Here's how the part is built. I have some questions about the finished solid (model axes, mm). Round coordinates to 2 decimals unless told otherwise and drop trailing zeros. Write each loop counter-clockwise with the first axis right and the second up, starting at its lowest first coordinate (ties: lowest second). Pieces come first, ordered by that corner, then holes. Notation, with made-up numbers: (35.5, 27.25) -> (69.5, 27.25) arc R19 cw to (69.5, 57.25) -> close; hole circle Ø7 at (-10, -3). An arc over 180 degrees is marked (long way). Answer as CSV lines item,"result".
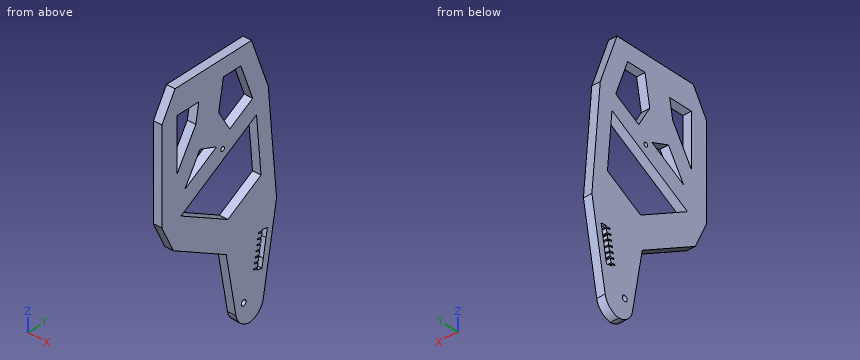
```python
from build123d import *

# Parameters (mm, degrees)
ESQUISSE1_W                             = 300
ESQUISSE1_H                             = 150
BOSS_EXTRU_1_DEPTH                      = 5
ESQUISSE2_OUTSIDE_W                     = 369.112
ESQUISSE2_OUTSIDE_H                     = 219.112
ENL_V_MAT_EXTRU_1_DEPTH                 = 5
ENL_V_MAT_EXTRU_2_DEPTH                 = 336.559234711
ENL_V_MAT_EXTRU_2_DEPTH_BACK            = 336.559234711
ENL_V_MAT_EXTRU_4_DEPTH                 = 336.559234711
ENL_V_MAT_EXTRU_4_DEPTH_BACK            = 336.559234711
ESQUISSE5_R                             = 3.2
EMPREINTE1_START                        = -213.565883238
EMPREINTE1_OUTLINE_W                    = 10
EMPREINTE1_OUTLINE_H                    = 6
EMPREINTE1_DEPTH                        = 20
D_PLACER_START                          = -213.815883238
D_PLACER_LA_FACE1_OUTLINE_W             = 10
D_PLACER_LA_FACE1_OUTLINE_H             = 6.5
D_PLACER_LA_FACE1_DEPTH                 = 20.5
D_PLACER_LA_FACE2_BY                    = 10
D_PLACER_LA_FACE3_BY                    = 10
ENL_V_MAT_EXTRU_5_DEPTH                 = 336.559234711
R_P_TITION_LIN_AIRE1_COUNT              = 7
R_P_TITION_LIN_AIRE1_PITCH              = 6
CONG_1_R                                = 20
PER_AGE_POUR_CROUS_AUTO_BLOQUANTS_300_D = 4.7625


# Read off the part's stored shape, not the designer's step: Empreinte1, Déplacer la face1
with BuildPart() as part:
    # Esquisse1 → Boss.-Extru.1 (new, symmetric)
    with BuildSketch(Plane(origin=(0, 0, 0), x_dir=(0, 0, -1), z_dir=(1, 0, 0))):
        with Locations((150, 75)):
            Rectangle(ESQUISSE1_W, ESQUISSE1_H)
    extrude(amount=BOSS_EXTRU_1_DEPTH, both=True)

    # Esquisse2 outside → Enlèv. mat.-Extru.1 (cut, symmetric)
    with BuildSketch(Plane(origin=(0, 0, 0), x_dir=(0, 0, -1), z_dir=(1, 0, 0))):
        with Locations((150, 75)):
            Rectangle(ESQUISSE2_OUTSIDE_W, ESQUISSE2_OUTSIDE_H)
        Polygon((0, 117.225703003), (60, 139.063917059), (185, 150), (300, 129.722397219), (300, 99.722397219), (211.741963761, 84.160124165), (171.741963761, 14.878091862), (139.835792798, 0), (29.835792798, 0), (0, 17.225703003), align=None, mode=Mode.SUBTRACT)
    extrude(amount=ENL_V_MAT_EXTRU_1_DEPTH, both=True, mode=Mode.SUBTRACT)

    # Esquisse3 → Enlèv. mat.-Extru.2 (cut, two sides: drawn at the far end of the back side and taken through both)
    with BuildSketch(Plane(origin=(5, 0, 0), x_dir=(0, 0, -1), z_dir=(1, 0, 0)).offset(-ENL_V_MAT_EXTRU_2_DEPTH_BACK)):
        Polygon((20, 103.221552239), (20, 80.493304508), (55, 74.321860183), (80, 88.755616913), (62.679491924, 118.755616913), align=None)
        Polygon((90, 71.435108837), (113.922571241, 30), (81.508057782, 49.831775443), align=None)
        Polygon((82.886751346, 123.755616913), (139.903333355, 25), (175.32640016, 86.354551467), (150.32640016, 129.655821657), align=None)
        Polygon((91.944969354, 20), (30, 20), (30, 48.267236345), (52.117107943, 44.367393479), align=None)
    extrude(amount=ENL_V_MAT_EXTRU_2_DEPTH + ENL_V_MAT_EXTRU_2_DEPTH_BACK, mode=Mode.SUBTRACT)

    # Esquisse5 → Enlèv. mat.-Extru.4 (cut, two sides: drawn at the far end of the back side and taken through both)
    with BuildSketch(Plane.ZY.offset(5).offset(-ENL_V_MAT_EXTRU_4_DEPTH_BACK)):
        with Locations((-275, 107.010571736)):
            Circle(ESQUISSE5_R)
    extrude(amount=ENL_V_MAT_EXTRU_4_DEPTH + ENL_V_MAT_EXTRU_4_DEPTH_BACK, mode=Mode.SUBTRACT)

    # Empreinte1 outline → Empreinte1 (cut)
    with BuildSketch(Plane(origin=(0, 0, 0), x_dir=(1, 0, 0), z_dir=(0, 0.173648177666931, 0.984807753012208)).offset(EMPREINTE1_START)):
        with Locations((0, 169.157749671)):
            Rectangle(EMPREINTE1_OUTLINE_W, EMPREINTE1_OUTLINE_H)
    extrude(amount=EMPREINTE1_DEPTH, mode=Mode.SUBTRACT)

    # Déplacer la face1 outline → Déplacer la face1 (cut)
    with BuildSketch(Plane(origin=(0, 0, 0), x_dir=(1, 0, 0), z_dir=(0, 0.173648177666931, 0.984807753012208)).offset(D_PLACER_START)):
        with Locations((0, 169.157749671)):
            Rectangle(D_PLACER_LA_FACE1_OUTLINE_W, D_PLACER_LA_FACE1_OUTLINE_H)
    extrude(amount=D_PLACER_LA_FACE1_DEPTH, mode=Mode.SUBTRACT)

    # Déplacer la face2: a face moved inward by 10.0
    extrude(part.faces().sort_by_distance((0, 133.01891252, -219.752915562))[0], amount=D_PLACER_LA_FACE2_BY, dir=(0, 0.173648178, 0.984807753), mode=Mode.SUBTRACT)

    # Déplacer la face3: a face moved inward by 10.0
    extrude(part.faces().sort_by_distance((0, 129.459124878, -239.941474499))[0], amount=D_PLACER_LA_FACE3_BY, dir=(0, -0.173648178, -0.984807753), mode=Mode.SUBTRACT)

    # Esquisse6 → Enlèv. mat.-Extru.5 (cut, through all)
    with BuildSketch(Plane(origin=(5, 0, 0), x_dir=(0, 0, -1), z_dir=(1, 0, 0))):
        Polygon((210.817693083, 131.294296833), (209.949452195, 126.370258067), (211.328183049, 126.127150619), (212.196423938, 131.051189384), align=None)
    enl_v_mat_extru_5 = extrude(amount=-ENL_V_MAT_EXTRU_5_DEPTH, mode=Mode.SUBTRACT)

    # Répétition linéaire1: Enlèv. mat.-Extru.5 ×7
    with Locations(*[Vector(0, -0.17364817766693066, -0.9848077530122081) * (i * R_P_TITION_LIN_AIRE1_PITCH) for i in range(1, R_P_TITION_LIN_AIRE1_COUNT)]):
        add(enl_v_mat_extru_5, mode=Mode.SUBTRACT)

    # Congé1
    # the kernel refuses this fillet: 20 mm, written as the material it takes off along each edge
    with BuildSketch(Plane(origin=(-46.954981559, 129.722397219, -300), x_dir=(0, 0.17364817766693125, 0.9848077530122079), z_dir=(1, 0, 0))) as cong_1_piece_1:
        with BuildLine():
            CenterArc((CONG_1_R * 0.839099631177, CONG_1_R), CONG_1_R, 190, 80)
            Line((-CONG_1_R * 0.145708121835, CONG_1_R * 0.826351822333), (0, 0))
            Line((0, 0), (CONG_1_R * 0.839099631177, 0))
        make_face()
    extrude(amount=93.909963118, mode=Mode.SUBTRACT)
    with BuildSketch(Plane(origin=(-46.954981559, 99.722397219, -300), x_dir=(0, -0.17364817766692434, 0.984807753012209), z_dir=(1, 0, 0))) as cong_1_piece_2:
        with BuildLine():
            CenterArc((CONG_1_R * 0.839099631177, -CONG_1_R), CONG_1_R, 90, 80)
            Line((-CONG_1_R * 0.145708121835, -CONG_1_R * 0.826351822333), (0, 0))
            Line((0, 0), (CONG_1_R * 0.839099631177, 0))
        make_face()
    extrude(amount=93.909963118, mode=Mode.SUBTRACT)

    # Perçage pour écrous auto-bloquants 300® #6 (SP)1 (through all)
    with Locations(Plane(origin=(5, 0, 0), x_dir=(0, 0, -1), z_dir=(1, 0, 0))):
        with Locations((96.461753504, 79.36920384)):
            Hole(PER_AGE_POUR_CROUS_AUTO_BLOQUANTS_300_D / 2)


solid = part.part
```
1. For pin 1 Ø1 at (x, z) = (2, -70.5) entering from -Y; pin 2 Ø5 at (x, z) = (1, -75.5) entering from +Y; pin 3 Ø1 at (x, z) = (-3.5, -136) entering from +Y, each with a flat end and sliding along its axis, tell me the tip position at first contact or that it passes through.
Numbers:
pin 1,"stops at y = 0"
pin 2,"stops at y = 140.64"
pin 3,"stops at y = 145.76"
2. Suppose I cut it at C-C on y = 38. Please give me the cut outline in (x, z), and give its area (3 significant figures).
Numbers:
outline,"(-5, -185.09) -> (5, -185.09) -> (5, -147.41) -> (-5, -147.41) -> close; (-5, -132.4) -> (5, -132.4) -> (5, -109.3) -> (-5, -109.3) -> close; (-5, -100.85) -> (5, -100.85) -> (5, -62.52) -> (-5, -62.52) -> close; (-5, -30) -> (5, -30) -> (5, 0) -> (-5, 0) -> close"
area,"1,290 mm^2"
3. Suppose I cut it at A-A on z = -275. Please give me the cut outline in (x, y).
Numbers:
outline,"(-5, 95.31) -> (5, 95.31) -> (5, 103.81) -> (-5, 103.81) -> close; (-5, 110.21) -> (5, 110.21) -> (5, 134.13) -> (-5, 134.13) -> close"
4. If I drill on line 1 (Z direction, x = -2, y = 53); line 2 (Z direction, x = -0.25, y = 98.5); line 3 (Y direction, x = 3, z = -231.5), over which ranges is the centre line in solid material (lowest first)?
Numbers:
line 1,"z = -193.75 to -156.07, -123.74 to -100.64, -82.75 to 0"
line 2,"z = -288.71 to -168.31, -97.47 to -74.37, -20 to 0"
line 3,"y = 87.64 to 127.65, 134.25 to 141.8"
5. Suppose I cut it at D-D on z = -166. Please give me the cut outline in (x, y).
Numbers:
outline,"(-5, 12.2) -> (5, 12.2) -> (5, 70.2) -> (-5, 70.2) -> close; (-5, 102.51) -> (5, 102.51) -> (5, 148.34) -> (-5, 148.34) -> close"
6. Suppose I cut it at B-B on y = 63. Please give me the cut outline in (x, z), and give its area (3 significant figures).
Numbers:
outline,"(-5, -199.53) -> (5, -199.53) -> (5, -161.84) -> (-5, -161.84) -> close; (-5, -117.96) -> (5, -117.96) -> (5, -94.87) -> (-5, -94.87) -> close; (-5, -86.68) -> (5, -86.68) -> (5, 0) -> (-5, 0) -> close"
area,"1,470 mm^2"
